Source: CAD feature listing. Evaluate the final solid. Frame: model axes, mm. Face numbers are marked on the shaded views. A direction names the side the tool comes from. Give positions to 0.01 mm unless a question says otherwise; leave off trailing zeros. Loops run counter-clockwise (first coordinate to the right, second up) from the corner with the lowest first, then second, coordinate; pieces in that order, holes last.
```python
from build123d import *

# Parameters (mm, degrees)
EXTRUDE_1_DEPTH     = 1
EXTRUDE_2_DEPTH     = 40
SKETCH_3_W          = 127.6
SKETCH_3_H          = 10
SKETCH_3_R          = 2
SKETCH_3_W_2        = 10
SKETCH_3_H_2        = 37
EXTRUDE_3_DEPTH     = 3
SKETCH_4_W          = 2
SKETCH_4_H          = 38.5
CUT_EXTRUDE_1_DEPTH = 176.951015911


with BuildPart() as part:
    # 草图1 → 凸台-拉伸1 (new body)
    with BuildSketch(Plane.XY):
        Polygon((-63.8, 104), (63.8, 104), (63.8, 36), (44.8, 36), (44.8, 0), (-44.8, 0), (-44.8, 36), (-63.8, 36), align=None)
    extrude(amount=EXTRUDE_1_DEPTH)

    # 草图2 → 凸台-拉伸2 (add)
    with BuildSketch(Plane.XY.offset(1)):
        Polygon((-44.8, 36), (-44.8, 0), (44.8, 0), (44.8, 36), (63.8, 36), (63.8, 104), (-63.8, 104), (-63.8, 36), align=None)
        Polygon((62.8, 103), (-62.8, 103), (-62.8, 37), (-43.8, 37), (-43.8, 1), (43.8, 1), (43.8, 37), (62.8, 37), align=None, mode=Mode.SUBTRACT)
    extrude(amount=EXTRUDE_2_DEPTH)

    # 草图3 → 凸台-拉伸3 (add)
    # profile 1 of 3: a face of its own
    with BuildSketch(Plane.XY.offset(41)):
        with Locations((0, 109)):
            Rectangle(SKETCH_3_W, SKETCH_3_H)
        with Locations((58.8, 109.5)):
            Circle(SKETCH_3_R, mode=Mode.SUBTRACT)
        with Locations(Location((-58.8, 109.5, 0), (0, 0, 180))):
            Circle(SKETCH_3_R, mode=Mode.SUBTRACT)
    # profile 2 of 3: a face of its own
    with BuildSketch(Plane.XY.offset(41)):
        with Locations((48.8, 18.5)):
            Rectangle(SKETCH_3_W_2, SKETCH_3_H_2)
        with Locations((50, 5)):
            Circle(SKETCH_3_R, mode=Mode.SUBTRACT)
    # profile 3 of 3: a face of its own
    with BuildSketch(Plane.XY.offset(41)):
        with Locations((-48.8, 18.5)):
            Rectangle(SKETCH_3_W_2, SKETCH_3_H_2)
        with Locations(Location((-50, 5, 0), (0, 0, 180))):
            Circle(SKETCH_3_R, mode=Mode.SUBTRACT)
    extrude(amount=-EXTRUDE_3_DEPTH)

    # 草图4 → 切除-拉伸1 (cut, through all)
    with BuildSketch(Plane.ZY.offset(63.8)):
        with Locations((40, 94.75)):
            Rectangle(SKETCH_4_W, SKETCH_4_H)
    extrude(amount=-CUT_EXTRUDE_1_DEPTH, mode=Mode.SUBTRACT)


solid = part.part
```
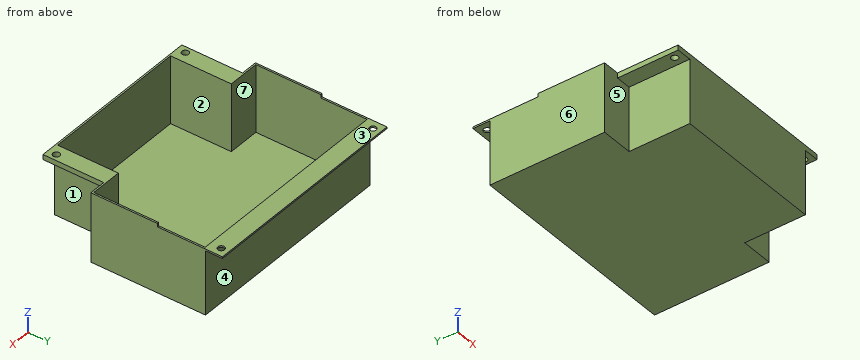
(1) Reachability of the marked faces 1, 2, 3 and 4 from +Z, -Z, +X, -X, +Y, -Y: full face, straight path, thin tool, end or side. Return the list, or none.
A:
face 1: -Z, +X, -Y
face 2: +Z
face 3: +Z, +X, -X, +Y
face 4: -Z, +X, -X, +Y
(2) Section B-B, the plane z = 3.5. Return the cut outline in (x, y), then the cut area to 3 significant figures.
A:
outline: (-63.8, 36) - (-44.8, 36) - (-44.8, 0) - (44.8, 0) - (44.8, 36) - (63.8, 36) - (63.8, 104) - (-63.8, 104) - close; hole (-62.8, 37) - (-43.8, 37) - (-43.8, 1) - (43.8, 1) - (43.8, 37) - (62.8, 37) - (62.8, 103) - (-62.8, 103) - close
area: 459 mm2
(3) Ray query, line 1 along Y through (x, z) = (-50, 38.75); line 2 along Y through (x, z) = (13, 11.5); line 3 along X through (y, z) = (30.5, 9). Return the intervals inside material, ascending.
A:
line 1: y = 0 to 3, 7 to 37, 103 to 114
line 2: y = 0 to 1, 103 to 104
line 3: x = -44.8 to -43.8, 43.8 to 44.8
(4) Mould query, pull axis X, two halves, no side actions, for the marked faces 5, 6 and 7. Classes: pulls with the +X half, pulls with the -X half, needs draft (parallel to the pull), parting line crosses it, or undercut.
A:
face 5: needs draft
face 6: pulls with the -X half
face 7: undercut
(5) Section D-D, the plane y = 89. Return the cut outline in (x, z).
A:
outline: (-63.8, 0) - (63.8, 0) - (63.8, 39) - (62.8, 39) - (62.8, 1) - (-62.8, 1) - (-62.8, 39) - (-63.8, 39) - close
(6) Section A-A, the plane y = 5. Return the cut outline in (x, z).
A:
outline: (-53.8, 38) - (-52, 38) - (-52, 41) - (-53.8, 41) - close; (-48, 38) - (-44.8, 38) - (-44.8, 0) - (44.8, 0) - (44.8, 38) - (48, 38) - (48, 41) - (43.8, 41) - (43.8, 1) - (-43.8, 1) - (-43.8, 41) - (-48, 41) - close; (52, 38) - (53.8, 38) - (53.8, 41) - (52, 41) - close
(7) Section C-C, the plane x = -58.8. Return the cut outline in (y, z), then the cut area to 3 significant figures.
A:
outline: (36, 0) - (104, 0) - (104, 38) - (107.5, 38) - (107.5, 39) - (103, 39) - (103, 1) - (37, 1) - (37, 41) - (36, 41) - close; (111.5, 38) - (114, 38) - (114, 39) - (111.5, 39) - close
area: 152 mm2
(8) First-contact query: pin 1 (6 mm diameter, centred on x = 2.5, y = 49, fed in from +Z); pin 2 (0.9 mm diameter, centred on y = 22.5, z = 39, fed in from +X); pin 3 (4 mm diameter, centred on x = 47, z = 7.5, fed in from +Y); pin 4 (2.5 mm diameter, centred on x = -50, y = 5, fed in from -Z) (3 decimals). Flat tips, straight axial feed; report the tip coordinate or a pass-through.
A:
pin 1: stops at z = 1
pin 2: stops at x = 53.8
pin 3: stops at y = 104
pin 4: passes through
